```python
from build123d import *

# Parameters (mm, degrees)
SKETCH1_R           = 12.5
BOSS_EXTRUDE1_DEPTH = 20
SKETCH1_4_R         = 12.5
SKETCH1_4_R_2       = 10
BOSS_EXTRUDE2_DEPTH = 13


with BuildPart() as part:
    # Sketch1 → Boss-Extrude1 (new body)
    with BuildSketch(Plane(origin=(0, 0, 0), x_dir=(1, 0, 0), z_dir=(0, 1, 0))):
        with BuildLine():
            ThreePointArc((37.5, 97.5), (30, 90), (37.5, 82.5))
            Line((37.5, 82.5), (50, 82.5))
            Line((50, 82.5), (50, 80))
            Line((50, 80), (30, 80))
            Line((30, 80), (30, 0))
            Line((30, 0), (0, 0))
            Line((0, 0), (0, 100))
            Line((0, 100), (50, 100))
            Line((50, 100), (50, 97.5))
            Line((50, 97.5), (37.5, 97.5))
        make_face()
        with Locations(Location((15, 15, 0), (0, 0, 270))):
            Circle(SKETCH1_R, mode=Mode.SUBTRACT)
    extrude(amount=BOSS_EXTRUDE1_DEPTH)

    # Sketch1_4 → Boss-Extrude2 (add)
    with BuildSketch(Plane(origin=(0, 0, 0), x_dir=(1, 0, 0), z_dir=(0, 1, 0))):
        with Locations(Location((15, 15, 0), (0, 0, 270))):
            Circle(SKETCH1_4_R)
        with Locations(Location((15, 15, 0), (0, 0, 90))):
            Circle(SKETCH1_4_R_2, mode=Mode.SUBTRACT)
    extrude(amount=BOSS_EXTRUDE2_DEPTH)


solid = part.part
```
Check sheet for the modelled part. Datum: model origin and axes. Units: mm. A direction names the side the tool comes from. Round coordinates to 2 decimals unless told otherwise and drop trailing zeros. Order: outer loops, then holes, each group sorted by start corner. A loop starts at its lowest first (then second) coordinate and runs counter-clockwise, first axis right, second up. Notation, with made-up numbers: M 86.25,53 L 92.25,53 A21 ccw 92.25,58 Z; hole C 64.25,-36 d3. An arc over 180 degrees is marked long. Answer in a Markdown table with one row per item.
(1) Section check D-D on x = 23. Record the boundary of the cut face in (y, z).
Findings:
| item | result |
|---|---|
| outline | M 0,-100 L 20,-100 L 20,-24.6 L 13,-24.6 L 13,-21 L 0,-21 Z; M 0,-9 L 13,-9 L 13,-5.4 L 20,-5.4 L 20,0 L 0,0 Z |
(2) Material ranges on line 1 along Z through (x, y) = (15.5, 7.5); line 2 along X through (y, z) = (9.5, -15); line 3 along X through (y, z) = (15.75, -15), recorded low to high. Write a range as from..to.
Findings:
| item | result |
|---|---|
| line 1 | z = -100..-24.99, -5.01..0 |
| line 2 | x = 0..5, 25..30 |
| line 3 | x = 0..2.5, 27.5..30 |
(3) Gauge pin test, flat ends, axial feed: pin 1 (4 mm diameter, centred on y = 14, z = -60.5, fed in from +X); pin 2 (6 mm diameter, centred on x = 45.5, y = 8, fed in from +Z); pin 3 (23 mm diameter, centred on x = 15, z = -15, fed in from +Y); pin 4 (15 mm diameter, centred on x = 15, z = -15, fed in from -Y). Record the tip position at first contact, or that the pin passes through.
Findings:
| item | result |
|---|---|
| pin 1 | stops at x = 30 |
| pin 2 | stops at z = -80 |
| pin 3 | stops at y = 13 |
| pin 4 | passes through |
(4) Section check C-C on x = 45. Record the boundary of the cut face in (y, z), plus the area to 3 significant figures.
Findings:
| item | result |
|---|---|
| outline | M 0,-100 L 20,-100 L 20,-97.5 L 0,-97.5 Z; M 0,-82.5 L 20,-82.5 L 20,-80 L 0,-80 Z |
| area | 100 mm^2 |
(5) Draft check along Z on faces 1 (the cylindrical face through (2.797, 16.451, -17.71)), 2 (the flat face through (30, 10, -41)), 3 (the flat face through (25.2, 13, -15.1)), 4 (the flat face through (15, 10, 0)). Enter one of: +Z half, -Z half, draft (parallel to the pull), parting line (faces both ways), or undercut.
Findings:
| item | result |
|---|---|
| face 1 | undercut |
| face 2 | draft |
| face 3 | undercut |
| face 4 | +Z half |
(6) Set-up check for faces 5 (the flat face through (40, 10, -80)), 6 (the flat face through (44, 10, -97.5)), 7 (the flat face through (25, 10, -100)): record each of +Z, -Z, +X, -X, +Y, -Y from which the full face is reachable in a straight line by a thin tool's end or side.
Findings:
| item | result |
|---|---|
| face 5 | +Z, +X, +Y, -Y |
| face 6 | +X, +Y, -Y |
| face 7 | -Z, +X, -X, +Y, -Y |
(7) Section check A-A on z = -15. Record the boundary of the cut face in (x, y).
Findings:
| item | result |
|---|---|
| outline | M 0,0 L 5,0 L 5,13 L 2.5,13 L 2.5,20 L 0,20 Z; M 25,0 L 30,0 L 30,20 L 27.5,20 L 27.5,13 L 25,13 Z |
(8) Section check B-B on y = 17. Record the boundary of the cut face in (x, z).
Findings:
| item | result |
|---|---|
| outline | M 0,-100 L 50,-100 L 50,-97.5 L 37.5,-97.5 A7.5 cw 37.5,-82.5 L 50,-82.5 L 50,-80 L 30,-80 L 30,0 L 0,0 Z; hole C 15,-15 d25 |
